```python
from build123d import *

# Parameters (mm, degrees)
SKETCH_1_R                  = 2.9
EXTRUDE_1_DEPTH             = 3.5
SKETCH_2_R                  = 2.5
EXTRUDE_2_DEPTH             = 10.5
CUT_EXTRUDE_1_DEPTH         = 4
HOLE_WIZARD_M32_D           = 2.8
HOLE_WIZARD_M32_DEPTH       = 6
HOLE_WIZARD_M32_CSINK_D     = 3.2
HOLE_WIZARD_M32_CSINK_ANGLE = 90
HOLE_WIZARD_M32_TIP         = 1.4


with BuildPart() as part:
    # Эскиз1 → Бобышка-Вытянуть1 (new body)
    with BuildSketch(Plane(origin=(0, 0, 0), x_dir=(1, 0, 0), z_dir=(0, 1, 0))):
        Circle(SKETCH_1_R)
    extrude(amount=EXTRUDE_1_DEPTH)

    # Эскиз2 → Бобышка-Вытянуть2 (add)
    with BuildSketch(Plane.XZ):
        Circle(SKETCH_2_R)
    extrude(amount=EXTRUDE_2_DEPTH)

    # Эскиз3 → Вырез-Вытянуть1 (cut)
    with BuildSketch(Plane(origin=(0, 3.5, 0), x_dir=(1, 0, 0), z_dir=(0, 1, 0))):
        Polygon((0, 2.55), (-0.366495157, 2.916495157), (0.366495157, 2.916495157), align=None)
        Polygon((0.634159212, 2.469887061), (0.370321814, 2.916011738), (1.080283889, 2.733724459), align=None)
        Polygon((1.228471869, 2.234582034), (1.083870103, 2.732304577), (1.726194412, 2.3791838), align=None)
        Polygon((1.74559512, 1.85887), (1.729314848, 2.37691667), (2.263641791, 1.875150272), align=None)
        Polygon((2.15303621, 1.366358327), (2.26610038, 1.872178348), (2.658856231, 1.253294157), align=None)
        Polygon((2.425194117, 0.787993336), (2.660498492, 1.249804175), (2.887004956, 0.55268896), align=None)
        Polygon((2.544968157, 0.160115825), (2.887727699, 0.548900209), (2.933752541, -0.182643716), align=None)
        Polygon((2.504832489, -0.477822352), (2.933510354, -0.186493176), (2.796161665, -0.906500217), align=None)
        Polygon((2.307308984, -1.085737193), (2.794969765, -0.910168509), (2.482877668, -1.573397974), align=None)
        Polygon((1.964808769, -1.625431174), (2.480810946, -1.576654607), (2.013585336, -2.141433351), align=None)
        Polygon((1.498852393, -2.062993336), (2.010773652, -2.144073698), (1.417772031, -2.574914594), align=None)
        Polygon((0.938717609, -2.370930039), (1.414392054, -2.576772752), (0.732874896, -2.846604484), align=None)
        Polygon((0.319599746, -2.529892488), (0.729139002, -2.847563698), (0.001928536, -2.939431745), align=None)
        Polygon((-0.319599746, -2.529892488), (-0.001928536, -2.939431745), (-0.729139002, -2.847563698), align=None)
        Polygon((-0.938717609, -2.370930039), (-0.732874896, -2.846604484), (-1.414392054, -2.576772752), align=None)
        Polygon((-1.498852393, -2.062993336), (-1.417772031, -2.574914594), (-2.010773652, -2.144073698), align=None)
        Polygon((-1.964808769, -1.625431174), (-2.013585336, -2.141433351), (-2.480810946, -1.576654607), align=None)
        Polygon((-2.307308984, -1.085737193), (-2.482877668, -1.573397974), (-2.794969765, -0.910168509), align=None)
        Polygon((-2.504832489, -0.477822352), (-2.796161665, -0.906500217), (-2.933510354, -0.186493176), align=None)
        Polygon((-2.544968157, 0.160115825), (-2.933752541, -0.182643716), (-2.887727699, 0.548900209), align=None)
        Polygon((-2.425194117, 0.787993336), (-2.887004956, 0.55268896), (-2.660498492, 1.249804175), align=None)
        Polygon((-2.15303621, 1.366358327), (-2.658856231, 1.253294157), (-2.26610038, 1.872178348), align=None)
        Polygon((-1.74559512, 1.85887), (-2.263641791, 1.875150272), (-1.729314848, 2.37691667), align=None)
        Polygon((-1.228471869, 2.234582034), (-1.726194412, 2.3791838), (-1.083870103, 2.732304577), align=None)
        Polygon((-0.634159212, 2.469887061), (-1.080283889, 2.733724459), (-0.370321814, 2.916011738), align=None)
    extrude(amount=-CUT_EXTRUDE_1_DEPTH, mode=Mode.SUBTRACT)

    # Сверло под метчик  спиральное M32
    with Locations(Plane(origin=(0, 3.5, 0), x_dir=(1, 0, 0), z_dir=(0, 1, 0))):
        with Locations((0, 0)):
            CounterSinkHole(HOLE_WIZARD_M32_D / 2, HOLE_WIZARD_M32_CSINK_D / 2, depth=HOLE_WIZARD_M32_DEPTH, counter_sink_angle=HOLE_WIZARD_M32_CSINK_ANGLE)
            with Locations((0, 0, -(HOLE_WIZARD_M32_DEPTH + HOLE_WIZARD_M32_TIP / 2))):  # 90° drill point
                Cone(0, HOLE_WIZARD_M32_D / 2, HOLE_WIZARD_M32_TIP, mode=Mode.SUBTRACT)


solid = part.part
```
Work out the finished part from the listing and answer in its coordinate system (mm). Give positions to 0.01 mm unless a question says otherwise; leave off trailing zeros. Loops run counter-clockwise (first coordinate to the right, second up) from the corner with the lowest first, then second, coordinate; pieces in that order, holes last. Notation, with made-up numbers: M 86,-13.75 L 128,-13.75 A19 cw 128,-1.75 Z; hole C 58,48.5 d4. An arc over 180 degrees is marked long. One line per item, written item: value. Start each with the question number.
1. Determine the mould class of faces 1 (the face through (-0.54, -5.18, -2.44)), 2 (the face through (1.4, 0.36, -0.06)), 3 (the face through (0, -10.5, 0)) for opening direction Z: released by +Z, released by -Z, zero draft, split by the parting line, or undercut.
2. Each of these flat-tipped pins is pushed along its axis until it touches: P1, Ø1.7, axis at x = 0, z = 0, coming from the +Y side; P2, Ø2, axis at x = 0, y = -1.5, coming from the -Z side; P3, Ø2, axis at x = 2, y = -8, coming from the +Z side. Where does it stop, or does it pass through?
3. Find section A-A (y = -0.75). Give the vertices of the cut face in (x, z), and give its area (3 significant figures).
4. Find section B-B (y = -8). Give the vertices of the cut face in (x, z).
5. Find the intervals of material crossed by probe 1 along Y at (x, z) = (-0.7, 2.45); probe 2 along Z at (x, y) = (-0.6, 2); probe 3 along X at (y, z) = (-2, 2), in increasing order.
Reported:
1. face 1: split by the parting line
1. face 2: undercut
1. face 3: zero draft
2. P1: stops at y = -3.05
2. P2: stops at z = -2.5
2. P3: stops at z = 2.29
3. outline: C 0,0 d5; hole C 0,0 d2.8
3. area: 13.5 mm²
4. outline: C 0,0 d5
5. probe 1: y = 0 to 3.5
5. probe 2: z = -2.53 to -1.26, 1.26 to 2.75
5. probe 3: x = -1.5 to 1.5
